from build123d import *

# Parameters (mm, degrees)
BOSS_EXTRUDE1_DEPTH = 5.9436
SKETCH3_R           = 4.7625
CUT_EXTRUDE1_DEPTH  = 6.9436
CUT_EXTRUDE2_DEPTH  = 6.9436
SKETCH5_W           = 50.8
SKETCH5_H           = 5.9436
BOSS_EXTRUDE2_DEPTH = 5.9436
SKETCH6_R           = 4.7625
CUT_EXTRUDE3_DEPTH  = 6.9436
SKETCH7_W           = 12.7
SKETCH7_H           = 97.7138
BOSS_EXTRUDE3_DEPTH = 5.9436
SKETCH8_R           = 1.1303
CUT_EXTRUDE4_DEPTH  = 6.9436


with BuildPart() as part:
    # Sketch1 → Boss-Extrude1 (new body)
    with BuildSketch(Plane.XY):
        Polygon((0, 0), (0, 97.7138), (35.9029, 97.7138), (135.6995, 173.228), (178.8287, 173.228), (178.8287, 0), align=None)
    extrude(amount=BOSS_EXTRUDE1_DEPTH)

    # Sketch3 → Cut-Extrude1 (cut, through all)
    with BuildSketch(Plane.XY.offset(5.9436)):
        with Locations((81.1149, 97.7138)):
            Circle(SKETCH3_R)
    extrude(amount=-CUT_EXTRUDE1_DEPTH, mode=Mode.SUBTRACT)

    # Sketch4 → Cut-Extrude2 (cut, through all)
    with BuildSketch(Plane.XY.offset(5.9436)):
        Polygon((12.7, 3.96875), (12.7, 0), (15.6464, 0), (15.6464, 3.96875), (17.3482, 3.96875), (17.3482, 6.35), (15.6464, 6.35), (15.6464, 12.7), (12.7, 12.7), (12.7, 6.35), (10.9982, 6.35), (10.9982, 3.96875), align=None)
        Polygon((87.94115, 3.96875), (87.94115, 0), (90.88755, 0), (90.88755, 3.96875), (92.58935, 3.96875), (92.58935, 6.35), (90.88755, 6.35), (90.88755, 12.7), (87.94115, 12.7), (87.94115, 6.35), (86.23935, 6.35), (86.23935, 3.96875), align=None)
        Polygon((156.8323, 3.96875), (156.8323, 0), (159.7787, 0), (159.7787, 3.96875), (161.4805, 3.96875), (161.4805, 6.35), (159.7787, 6.35), (159.7787, 12.7), (156.8323, 12.7), (156.8323, 6.35), (155.1305, 6.35), (155.1305, 3.96875), align=None)
    extrude(amount=-CUT_EXTRUDE2_DEPTH, mode=Mode.SUBTRACT)

    # Sketch5 → Boss-Extrude2 (add)
    with BuildSketch(Plane.XY.offset(5.9436)):
        with Locations((51.793775, -2.9718)):
            Rectangle(SKETCH5_W, SKETCH5_H)
    extrude(amount=-BOSS_EXTRUDE2_DEPTH)

    # Sketch6 → Cut-Extrude3 (cut, through all)
    with BuildSketch(Plane.XY.offset(5.9436)):
        with Locations((81.1149, 65.9638)):
            Circle(SKETCH6_R)
    extrude(amount=-CUT_EXTRUDE3_DEPTH, mode=Mode.SUBTRACT)

    # Sketch7 → Boss-Extrude3 (add)
    with BuildSketch(Plane.XY.offset(5.9436)):
        with Locations((-6.35, 48.8569)):
            Rectangle(SKETCH7_W, SKETCH7_H)
    extrude(amount=-BOSS_EXTRUDE3_DEPTH)

    # Sketch8 → Cut-Extrude4 (cut, through all)
    with BuildSketch(Plane.XY.offset(5.9436)):
        with Locations((39.1414, 6.35)):
            Circle(SKETCH8_R)
        with Locations((172.4787, 6.35)):
            Circle(SKETCH8_R)
        with Locations((21.2344, 6.35)):
            Circle(SKETCH8_R)
    extrude(amount=-CUT_EXTRUDE4_DEPTH, mode=Mode.SUBTRACT)


solid = part.part
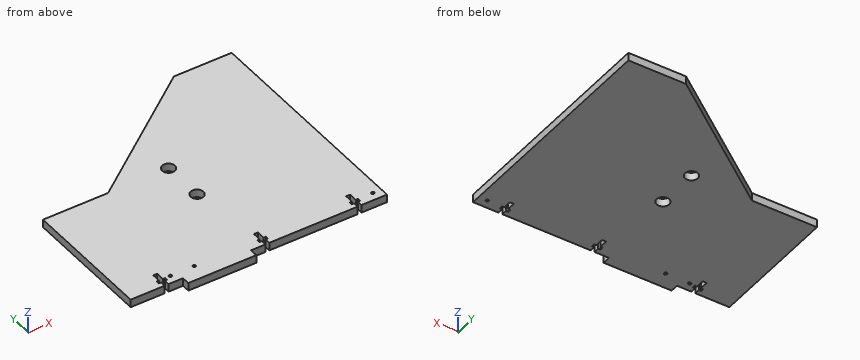
Here's how the part is built. I have some questions about the finished solid (model axes, mm). Round coordinates to 2 decimals unless told otherwise and drop trailing zeros. Write each loop counter-clockwise with the first axis right and the second up, starting at its lowest first coordinate (ties: lowest second). Pieces come first, ordered by that corner, then holes.
1. Suppose I cut it at A-A (y = 150). List the corners of the cut face in (x, z) for me, and give its area (3 significant figures).
2. I need wall thicknesses on L1, parallel to X at y = 97.5, z = 0.8; L2, parallel to Y at x = 24, z = 0.8; L3, parallel to X at y = 123, z = 3.3. Which ranges of each line are inside material? Lowest first, please.
3. Suppose I cut it at B-B (z = 3.45). State how many separate pieces and enclosed holes the cut face has, and give its area (3 significant figures).
4. Will these pins go through, and if not, where does the flat tip stop? pin 1 Ø3 at (x, z) = (125.5, 4) entering from -Y; pin 2 Ø2 at (x, z) = (61.5, 1) entering from +Y; pin 3 Ø0.5 at (x, z) = (16.5, 4) entering from +Y; pin 4 Ø10 at (x, y) = (134, 92.5) entering from -Z.
5. Suppose I cut it at C-C (x = 97). List the corners of the cut face in (y, z) for me, and give its area (3 significant figures).
Answer sheet:
1. outline: (105, 0) - (178.83, 0) - (178.83, 5.94) - (105, 5.94) - close
1. area: 439 mm2
2. L1: x = -12.7 to 76.36, 85.87 to 178.83
2. L2: y = 0 to 97.71
2. L3: x = 69.32 to 178.83
3. separate pieces: 1
3. enclosed holes: 5
3. area: 25,800 mm2
4. pin 1: stops at y = 0
4. pin 2: stops at y = 117.84
4. pin 3: stops at y = 97.71
4. pin 4: stops at z = 0
5. outline: (0, 0) - (143.94, 0) - (143.94, 5.94) - (0, 5.94) - close
5. area: 856 mm2
